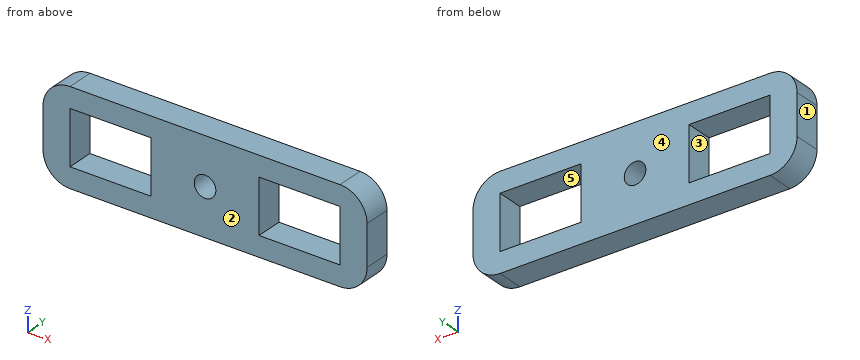
```python
from build123d import *

# Parameters (mm, degrees)
SKETCH1_R           = 4
SKETCH1_W           = 30
SKETCH1_H           = 20
BOSS_EXTRUDE1_DEPTH = 10


with BuildPart() as part:
    # Sketch1 → Boss-Extrude1 (new body)
    with BuildSketch(Plane(origin=(0, 0, 0), x_dir=(1, 0, 0), z_dir=(0, 1, 0))):
        with BuildLine():
            Line((10, 0), (110, 0))
            ThreePointArc((110, 0), (117.071067812, 2.928932188), (120, 10))
            Line((120, 10), (120, 25))
            ThreePointArc((120, 25), (117.071067812, 32.071067812), (110, 35))
            Line((110, 35), (10, 35))
            ThreePointArc((10, 35), (2.928932188, 32.071067812), (0, 25))
            Line((0, 25), (0, 10))
            ThreePointArc((0, 10), (2.928932188, 2.928932188), (10, 0))
        make_face()
        with Locations((60, 17.5)):
            Circle(SKETCH1_R, mode=Mode.SUBTRACT)
        with Locations((25, 17.5)):
            Rectangle(SKETCH1_W, SKETCH1_H, mode=Mode.SUBTRACT)
        with Locations((95, 17.5)):
            Rectangle(SKETCH1_W, SKETCH1_H, mode=Mode.SUBTRACT)
    extrude(amount=BOSS_EXTRUDE1_DEPTH)


solid = part.part
```
Read the model definition and answer for the solid it produces. Units are mm, in the model's axes. Face numbers are marked on the shaded views. A direction names the side the tool comes from. Give positions to 0.01 mm unless a question says otherwise; leave off trailing zeros. Loops run counter-clockwise (first coordinate to the right, second up) from the corner with the lowest first, then second, coordinate; pieces in that order, holes last.
Item 1: The part is cut by section C-C (y = 2.5). Write down the section's boundary in (x, z).
Item 2: The part is cut by section B-B (z = -17.5). Write down the section's boundary in (x, y), and give its area (3 significant figures).
Item 3: Each of these flat-tipped pins is pushed along its axis until it touches: pin 1 Ø1 at (x, z) = (66, -30) entering from -Y; pin 2 Ø5 at (y, z) = (6.5, -5.5) entering from +X. Where does it stop, or does it pass through?
Item 4: Find the intervals of material crossed by line 1 along X through (y, z) = (1, -24); line 2 along X through (y, z) = (4.75, -17.5); line 3 along Z through (x, y) = (60, 4.25), in increasing order.
Item 5: The part is cut by section A-A (x = 99). Write down the section's boundary in (y, z).
Item 6: For the marked faces 4 and 5, determine the directions among +Z, -Z, +X, -X, +Y, -Y from which every point of the face is accessible in a straight line to the end or side of a thin tool.
Item 7: The part is cut by section D-D (x = 60). Write down the section's boundary in (y, z), and give its area (3 significant figures).
Item 8: The mould has two halves that part along X. Classify the marked faces 1, 2 and 3: released by +X, released by -X, zero draft, split by the parting line, or undercut.
Taken from the geometry:
1. outline: (0, -25) arc R10 ccw to (10, -35) - (110, -35) arc R10 ccw to (120, -25) - (120, -10) arc R10 ccw to (110, 0) - (10, 0) arc R10 ccw to (0, -10) - close; hole (10, -27.5) - (40, -27.5) - (40, -7.5) - (10, -7.5) - close; hole circle Ø8 at (60, -17.5); hole (80, -27.5) - (110, -27.5) - (110, -7.5) - (80, -7.5) - close
2. outline: (0, 0) - (10, 0) - (10, 10) - (0, 10) - close; (40, 0) - (56, 0) - (56, 10) - (40, 10) - close; (64, 0) - (80, 0) - (80, 10) - (64, 10) - close; (110, 0) - (120, 0) - (120, 10) - (110, 10) - close
2. area: 520 mm2
3. pin 1: stops at y = 0
3. pin 2: stops at x = 119.8
4. line 1: x = 0 to 10, 40 to 80, 110 to 120
4. line 2: x = 0 to 10, 40 to 56, 64 to 80, 110 to 120
4. line 3: z = -35 to -21.5, -13.5 to 0
5. outline: (0, -35) - (10, -35) - (10, -27.5) - (0, -27.5) - close; (0, -7.5) - (10, -7.5) - (10, 0) - (0, 0) - close
6. face 4: +Z, -Z, +X, -X, +Y
6. face 5: +Y, -Y
7. outline: (0, -35) - (10, -35) - (10, -21.5) - (0, -21.5) - close; (0, -13.5) - (10, -13.5) - (10, 0) - (0, 0) - close
7. area: 270 mm2
8. face 1: released by -X
8. face 2: zero draft
8. face 3: undercut
